Here's how the part is built. I have some questions about the finished solid (model axes, mm). Face numbers are marked on the shaded views. A direction names the side the tool comes from. Round coordinates to 2 decimals unless told otherwise and drop trailing zeros. Order: outer loops, then holes, each group sorted by start corner. A loop starts at its lowest first (then second) coordinate and runs counter-clockwise, first axis right, second up. Notation, with made-up numbers: M -24.75,53.25 L -3.75,53.25 A21 cw -3.75,81.25 Z; hole C 28,-33 d6. An arc over 180 degrees is marked long. Write item = value, one per line. Start each with the question number.
Item 1: I want a section at A-A, the plane y = 0. List the corners of the cut face in (x, z) for me, plus the area to 3 significant figures.
Item 2: I want a section at B-B, the plane z = -1.5. List the corners of the cut face in (x, y) for me, plus the area to 3 significant figures.
Item 3: I'm going to push flat-ended pins straight in: P1, Ø10, axis at y = -12.5, z = 1.5, coming from the -X side; P2, Ø2.5, axis at x = 6.5, z = -12.5, coming from the +Y side; P3, Ø12, axis at y = 39.5, z = -5, coming from the +X side. Where does each tip first touch, or does it pass through?
Item 4: For the marked faces 5, 6 and 7, which set-ups out of +Z, -Z, +X, -X, +Y, -Y let a thin tool reach every point of the face, with its end or its side?
Item 5: We'd pull the mould along X, two halves only. Please class the marked faces 1, 2, 3 and 4: pulls with the +X half, pulls with the -X half, needs draft (parallel to the pull), parting line crosses it, or undercut.
Item 6: Please list where these lines run through material, in increasing order: L1, parallel to Z at x = 28, y = -2.5; L2, parallel to Z at x = 27.5, y = 22; L3, parallel to Z at x = -6.5, y = -7.5.
Item 7: I want a section at C-C, the plane z = -10. List the corners of the cut face in (x, y) for me, plus the area to 3 significant figures.
```python
from build123d import *

# Parameters (mm, degrees)
ESQUISSE1_R                  = 9.5
ESQUISSE1_R_2                = 6.35
BOSS_EXTRU_1_DEPTH           = 14.25
ENL_V_MAT_EXTRU_1_DEPTH      = 6
ENL_V_MAT_EXTRU_2_DEPTH      = 7.25
ENL_V_MAT_EXTRU_2_DEPTH_BACK = 7.25
ENL_V_MAT_EXTRU_3_DEPTH      = 5
ENL_V_MAT_EXTRU_3_DRAFT      = -5


with BuildPart() as part:
    # Esquisse1 → Boss.-Extru.1 (new, symmetric)
    with BuildSketch(Plane.XY):
        with BuildLine():
            Line((-26.61523279, 45.963348263), (-21.894870769, -2.148169925))
            ThreePointArc((-21.894870769, -2.148169925), (-14.777351956, -16.298155392), (0, -22))
            Line((0, -22), (59, -22))
            Line((59, -22), (59, -6.5))
            Line((59, -6.5), (37, -6.5))
            ThreePointArc((37, -6.5), (30.5, 0), (37, 6.5))
            Line((37, 6.5), (59, 6.5))
            Line((59, 6.5), (59, 14))
            ThreePointArc((59, 14), (23.937620364, 25.155899787), (0.053417306, 53.144636986))
            ThreePointArc((0.053417306, 53.144636986), (-16.322360933, 60.848824799), (-26.61523279, 45.963348263))
        make_face()
        with Locations(Location((0, 0, 0), (0, 0, 180))):
            Circle(ESQUISSE1_R, mode=Mode.SUBTRACT)
        with Locations(Location((-12.68213321, 47.330365488, 0), (0, 0, 180))):
            Circle(ESQUISSE1_R_2, mode=Mode.SUBTRACT)
    extrude(amount=BOSS_EXTRU_1_DEPTH, both=True)

    # Esquisse2 → Enlèv. mat.-Extru.1 (cut)
    with BuildSketch(Plane.XY.offset(14.25)):
        with BuildLine():
            Line((4.051067321, 38.330365488), (9.321809703, 38.330365488))
            ThreePointArc((9.321809703, 38.330365488), (4.202566317, 45.434036591), (0.053417306, 53.144636986))
            ThreePointArc((0.053417306, 53.144636986), (-16.322360933, 60.848824799), (-26.61523279, 45.963348263))
            Line((-26.61523279, 45.963348263), (-25.360971776, 33.179497931))
            ThreePointArc((-25.360971776, 33.179497931), (-9.404585059, 28.615193084), (4.051067321, 38.330365488))
        make_face()
    enl_v_mat_extru_1 = extrude(amount=-ENL_V_MAT_EXTRU_1_DEPTH, mode=Mode.SUBTRACT)

    # Symétrie1: Enlèv. mat.-Extru.1 across plane
    add(enl_v_mat_extru_1.mirror(Plane.XY), mode=Mode.SUBTRACT)

    # Esquisse3 → Enlèv. mat.-Extru.2 (cut, two sides: drawn at the far end of the back side and taken through both)
    with BuildSketch(Plane.XY.offset(-ENL_V_MAT_EXTRU_2_DEPTH_BACK)):
        with BuildLine():
            Line((21, -22), (21, 27.222240802))
            ThreePointArc((21, 27.222240802), (38.984037644, 17.691299917), (59, 14))
            Line((59, 14), (59, -22))
            Line((59, -22), (21, -22))
        make_face()
    extrude(amount=ENL_V_MAT_EXTRU_2_DEPTH + ENL_V_MAT_EXTRU_2_DEPTH_BACK, mode=Mode.SUBTRACT)


with BuildPart() as enl_v_mat_extru_3_tool:
    # Esquisse4 → Enlèv. mat.-Extru.3 (with draft: the straight prism first)
    with BuildSketch(Plane.XY.offset(14.25)):
        with BuildLine():
            Line((8.387524958, 36.330365488), (5.20641061, 36.330365488))
            ThreePointArc((5.20641061, 36.330365488), (-7.394798321, 27.006879326), (-22.942022259, 29.007301424))
            Line((-22.942022259, 29.007301424), (-19.904427971, -1.95288175))
            ThreePointArc((-19.904427971, -1.95288175), (-13.433956323, -14.816504902), (0, -20))
            Line((0, -20), (57, -20))
            Line((57, -20), (57, -8.5))
            Line((57, -8.5), (37, -8.5))
            ThreePointArc((37, -8.5), (28.5, 0), (37, 8.5))
            Line((37, 8.5), (57, 8.5))
            Line((57, 8.5), (57, 12.086242091))
            ThreePointArc((57, 12.086242091), (30.207518708, 19.223076596), (8.387524958, 36.330365488))
        make_face()
    extrude(amount=-ENL_V_MAT_EXTRU_3_DEPTH)
    # Enlèv. mat.-Extru.3: the draft: its side faces are tilted about the plane it starts from
    enl_v_mat_extru_3_sides = [enl_v_mat_extru_3_tool.faces().sort_by_distance(p)[0] for p in [
        (6.796967784, 36.330365488, 11.75),
        (-7.394798321, 27.006879326, 11.75),
        (-21.423225115, 13.527209837, 11.75),
        (-13.433956323, -14.816504902, 11.75),
        (28.5, -20, 11.75),
        (57, -14.25, 11.75),
        (47, -8.5, 11.75),
        (28.5, 0, 11.75),
        (47, 8.5, 11.75),
        (57, 10.293121046, 11.75),
        (30.207518708, 19.223076596, 11.75),
    ]]
    draft(enl_v_mat_extru_3_sides, Plane.XY.offset(14.25), ENL_V_MAT_EXTRU_3_DRAFT)


with BuildPart() as part_1:
    add(part.part)

    # Enlèv. mat.-Extru.3: cut by enl_v_mat_extru_3_tool
    add(enl_v_mat_extru_3_tool.part, mode=Mode.SUBTRACT)


solid = part_1.part
```
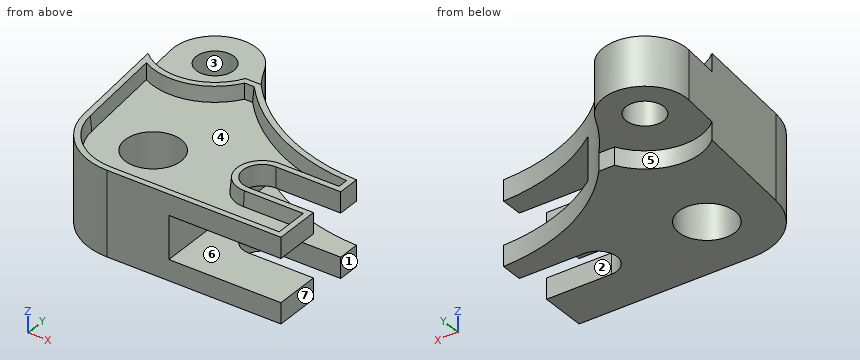
Filled in:
q1.outline = M -22.11,-14.25 L -9.5,-14.25 L -9.5,9.25 L -19.66,9.25 L -20.1,14.25 L -22.11,14.25 Z; M 9.5,-14.25 L 30.5,-14.25 L 30.5,-7.25 L 21,-7.25 L 21,7.25 L 30.5,7.25 L 30.5,14.25 L 28.5,14.25 L 28.06,9.25 L 9.5,9.25 Z
q1.area = 674 mm^2
q2.outline = M -26.62,45.96 L -21.89,-2.15 A22 ccw 0,-22 L 21,-22 L 21,27.22 A67 cw 0.05,53.14 A14 ccw Z; hole C -12.68,47.33 d12.7; hole C 0,0 d19
q2.area = 2,690 mm^2
q3.P1 = -20.68
q3.P2 = 38.33
q3.P3 = 13.72
q4.face_5 = -Z, +Y
q4.face_6 = +X, +Y, -Y
q4.face_7 = +Z, -Z, +X, +Y, -Y
q5.face_1 = pulls with the +X half
q5.face_2 = needs draft
q5.face_3 = undercut
q5.face_4 = undercut
q6.L1 = -14.25 to -7.25, 7.25 to 9.25
q6.L2 = -14.25 to -7.25, 7.25 to 14.25
q6.L3 = -14.25 to 9.25
q7.outline = M -25.36,33.18 L -21.89,-2.15 A22 ccw 0,-22 L 59,-22 L 59,-6.5 L 37,-6.5 A6.5 cw 37,6.5 L 59,6.5 L 59,14 A67 cw 9.32,38.33 L 4.05,38.33 A19 cw Z; hole C 0,0 d19
q7.area = 3,170 mm^2
